from build123d import *

# Parameters (mm, degrees)
F0_W     = 50.8
F0_H     = 25.4
F1_DEPTH = 19.05
F2_D     = 19.05
F4_D     = 6.35


with BuildPart() as f1:
    # F0 (on Front) → F1 (new body)
    with BuildSketch(Plane.XZ):
        Rectangle(F0_W, F0_H)
        with BuildLine():
            ThreePointArc((25.4, -12.7), (38.1, 0), (25.4, 12.7))
            Line((25.4, 12.7), (25.4, -12.7))
        make_face()
        with BuildLine():
            Line((-25.4, 12.7), (25.4, 12.7))
            ThreePointArc((25.4, 12.7), (0, 15.875), (-25.4, 12.7))
        make_face()
        with BuildLine():
            Line((-25.4, -12.7), (-25.4, 12.7))
            ThreePointArc((-25.4, 12.7), (-38.1, 0), (-25.4, -12.7))
        make_face()
        with BuildLine():
            ThreePointArc((-25.4, -12.7), (0, -15.875), (25.4, -12.7))
            Line((25.4, -12.7), (-25.4, -12.7))
        make_face()
    extrude(amount=F1_DEPTH)

    # F2 (through all)
    with Locations(Plane(origin=(0, 0, 0), x_dir=(1, 0, 0), z_dir=(0, 1, 0))):
        with Locations((0, 0)):
            Hole(F2_D / 2)

    # F4 (through all)
    with Locations(Plane.XZ.offset(19.05)):
        with Locations((-25.4, 0), (25.4, 0)):
            Hole(F4_D / 2)


solid = f1.part
For this review, take the finished solid that the model builds, in its own axes (mm). Give positions to 0.01 mm unless a question says otherwise; leave off trailing zeros. Loops run counter-clockwise (first coordinate to the right, second up) from the corner with the lowest first, then second, coordinate; pieces in that order, holes last. Notation, with made-up numbers: (1.25, -8) -> (12.25, -8) arc R27 ccw to (12.25, 8) -> close; hole circle Ø1 at (24, 26). An arc over 180 degrees is marked (long way). One line per question, with ' | ' between items.
1) Insertion check: pin 1 Ø4 at (y, z) = (-7.5, -8) entering from -X; pin 2 Ø5 at (y, z) = (-4, -8) entering from +X; pin 3 Ø1 at (x, y) = (-19.5, -5.5) entering from +Z; pin 4 Ø1 at (x, z) = (-7.5, -3.5) entering from +Y. Each pin has a flat end and moves straight along its axis. Give the tip position at first contact, or say it passes through.
Resolved:
pin 1: stops at x = -36.59 | pin 2: stops at x = 36.85 | pin 3: stops at z = 14.11 | pin 4: passes through
2) We need section A-A (z = 0). Write out the cut boundary in (x, y) (3 decimals), plus the area to 3 significant figures.
Resolved:
outline: (-38.1, -19.05) -> (-28.575, -19.05) -> (-28.575, 0) -> (-38.1, 0) -> close; (-22.225, -19.05) -> (-9.525, -19.05) -> (-9.525, 0) -> (-22.225, 0) -> close; (9.525, -19.05) -> (22.225, -19.05) -> (22.225, 0) -> (9.525, 0) -> close; (28.575, -19.05) -> (38.1, -19.05) -> (38.1, 0) -> (28.575, 0) -> close | area: 847 mm2
3) We need section D-D (z = -4.5). Write out the cut boundary in (x, y), plus the area to 3 significant figures.
Resolved:
outline: (-37.28, -19.05) -> (-8.39, -19.05) -> (-8.39, 0) -> (-37.28, 0) -> close; (8.39, -19.05) -> (37.28, -19.05) -> (37.28, 0) -> (8.39, 0) -> close | area: 1,100 mm2
4) To check wall thickness, follow probe 1 along Z at (x, y) = (25.4, -3.75) (3 decimals); probe 2 along X at (y, z) = (-14, 1.5); probe 3 along X at (y, z) = (-8, -4.5). State the ranges of each line that lie inside material, in increasing order.
Resolved:
probe 1: z = -12.7 to -3.175, 3.175 to 12.7 | probe 2: x = -38.01 to -28.2, -22.6 to -9.41, 9.41 to 22.6, 28.2 to 38.01 | probe 3: x = -37.28 to -8.39, 8.39 to 37.28
5) We need section C-C (y = -12.25). Give the number of separate pieces and of enclosed holes in the cut face, plus the area to 3 significant figures.
Resolved:
separate pieces: 1 | enclosed holes: 3 | area: 1,660 mm2
6) The part is to be moulded in two halves that separate along Z. For faces 1 (the cylindrical face through (-28.43, -9.39, 0.95)), 2 (the cylindrical face through (7.559, -9.658, 5.796)), 3 (the cylindrical face through (38.097, -9.392, -0.279)), 4 (the flat face through (-9, -19.05, 4)), say which applies: +Z half, -Z half, draft (parallel to the pull), parting line (faces both ways), or undercut.
Resolved:
face 1: undercut | face 2: undercut | face 3: parting line | face 4: draft
7) We need section B-B (x = 0). Write out the cut boundary in (y, z) (3 decimals).
Resolved:
outline: (-19.05, -15.875) -> (0, -15.875) -> (0, -9.525) -> (-19.05, -9.525) -> close; (-19.05, 9.525) -> (0, 9.525) -> (0, 15.875) -> (-19.05, 15.875) -> close
